Here's how the part is built. I have some questions about the finished solid (model axes, mm). Face numbers are marked on the shaded views. A direction names the side the tool comes from. Coordinates: 2 decimals unless noted, no trailing zeros. Loops run counter-clockwise (first coordinate to the right, second up) from the corner with the lowest first, then second, coordinate; pieces in that order, holes last. Notation, with made-up numbers: (6, -34.5) -> (11, -34.5) arc R26 cw to (11, -1.5) -> close; hole circle Ø10 at (42, -38.5). An arc over 180 degrees is marked (long way). Use CSV: the item, a comma, the result in double quotes. Start each with the question number.
from build123d import *

# Parameters (mm, degrees)
SKETCH1_W           = 127
SKETCH1_H           = 76.2
BOSS_EXTRUDE1_DEPTH = 76.2
CUT_EXTRUDE1_DEPTH  = 77.2
SKETCH3_W           = 58.776435242
SKETCH3_H           = 37.074512471
CUT_EXTRUDE2_DEPTH  = 77.2
SKETCH4_W           = 49.167351348
SKETCH4_H           = 86.931479723
BOSS_EXTRUDE3_DEPTH = 37.074512
CHAMFER1_SIZE       = 5.08
SKETCH5_R           = 3.175
BOSS_EXTRUDE4_DEPTH = 12.7
SKETCH6_W           = 49.167351348
SKETCH6_H           = 37.84167341
BOSS_EXTRUDE5_DEPTH = 5.08
SKETCH7_W           = 12.7
SKETCH7_H           = 3.957251341
BOSS_EXTRUDE6_DEPTH = 50.8
CHAMFER2_SIZE       = 4.445


with BuildPart() as part:
    # Sketch1 → Boss-Extrude1 (new body)
    with BuildSketch(Plane(origin=(0, 0, 0), x_dir=(1, 0, 0), z_dir=(0, 1, 0))):
        with Locations((63.5, 38.1)):
            Rectangle(SKETCH1_W, SKETCH1_H)
    extrude(amount=BOSS_EXTRUDE1_DEPTH)

    # Sketch2 → Cut-Extrude1 (cut, through all)
    with BuildSketch(Plane(origin=(0, 76.2, 0), x_dir=(1, 0, 0), z_dir=(0, 1, 0))):
        Polygon((86.341048303, 0), (105.391048303, 0), (105.391048303, 6.858), (111.233048303, 12.7), (80.499048303, 12.7), (86.341048303, 6.858), align=None)
    extrude(amount=-CUT_EXTRUDE1_DEPTH, mode=Mode.SUBTRACT)

    # Sketch3 → Cut-Extrude2 (cut, through all)
    with BuildSketch(Plane(origin=(0, 0, -76.2), x_dir=(-1, 0, 0), z_dir=(0, 0, -1))):
        with Locations((-29.388217621, 57.662743765)):
            Rectangle(SKETCH3_W, SKETCH3_H)
    extrude(amount=-CUT_EXTRUDE2_DEPTH, mode=Mode.SUBTRACT)

    # Sketch4 → Boss-Extrude3 (add)
    with BuildSketch(Plane(origin=(0, 39.125487529, 0), x_dir=(1, 0, 0), z_dir=(0, 1, 0))):
        with Locations((29.732558923, -5.365739861)):
            Rectangle(SKETCH4_W, SKETCH4_H)
    extrude(amount=BOSS_EXTRUDE3_DEPTH)

    # Chamfer1
    chamfer1_edges = [part.edges().sort_by_distance(p)[0] for p in [
        (5.148883249, 76.199999529, 5.365739861),
        (5.148883249, 39.125487529, 24.415739861),
        (54.316234597, 76.199999529, 5.365739861),
        (54.316234597, 39.125487529, 24.415739861),
    ]]
    chamfer(chamfer1_edges, length=CHAMFER1_SIZE)

    # Sketch5 → Boss-Extrude4 (add)
    with BuildSketch(Plane(origin=(0, 0, -38.1), x_dir=(-1, 0, 0), z_dir=(0, 0, -1))):
        with Locations((-45.312372158, 67.135265035)):
            Circle(SKETCH5_R)
        with Locations((-15.471955986, 67.135265035)):
            Circle(SKETCH5_R)
        with Locations((-45.312372158, 45.448629278)):
            Circle(SKETCH5_R)
        with Locations((-15.471955986, 45.448629278)):
            Circle(SKETCH5_R)
    extrude(amount=BOSS_EXTRUDE4_DEPTH)

    # Sketch6 → Boss-Extrude5 (add)
    with BuildSketch(Plane(origin=(0, 0, -50.8), x_dir=(-1, 0, 0), z_dir=(0, 0, -1))):
        with Locations((-29.732558923, 58.046324234)):
            Rectangle(SKETCH6_W, SKETCH6_H)
    extrude(amount=BOSS_EXTRUDE5_DEPTH)

    # Sketch7 → Boss-Extrude6 (add)
    with BuildSketch(Plane(origin=(0, 0, -55.88), x_dir=(-1, 0, 0), z_dir=(0, 0, -1))):
        with Locations((-40.016034597, 43.1361132)):
            Rectangle(SKETCH7_W, SKETCH7_H)
        with Locations((-19.365834597, 43.1361132)):
            Rectangle(SKETCH7_W, SKETCH7_H)
    extrude(amount=BOSS_EXTRUDE6_DEPTH)

    # Chamfer2
    chamfer2_edges = [part.edges().sort_by_distance(p)[0] for p in [
        (46.366034597, 43.1361132, -106.68),
        (33.666034597, 43.1361132, -106.68),
        (25.715834597, 43.1361132, -106.68),
        (13.015834597, 43.1361132, -106.68),
    ]]
    chamfer(chamfer2_edges, length=CHAMFER2_SIZE)


solid = part.part
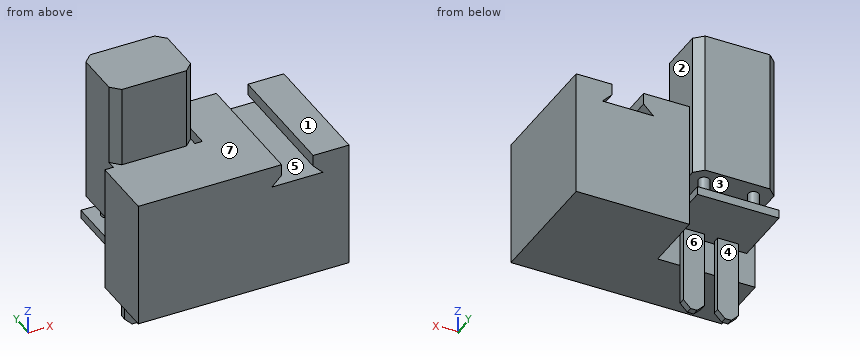
1) Which directions (+Z, -Z, +X, -X, +Y, -Y) give clear straight access to the entire face, cutting with the end or side of a thin tool? Please do the marked faces 1, 2, 3 and 4.
2) Please list where these lines run through material, in increasing order: L1, parallel to Z at x = 9, y = 48; L2, parallel to Y at x = 36.5, z = -67; L3, parallel to X at y = 31, z = -3.5. Write a range as [from, to].
3) I want a section at B-B, the plane y = 52.5. Please give me the cut outline in (x, z), plus the area to 3 significant figures.
4) I want a section at A-A, the plane z = -95.5. Please give me the cut outline in (x, y), plus the area to 3 significant figures.
5) Thinking about a two-plate mould opening in Z: for the marked faces 5, 6 and 7, which applies, pulls with the +Z half, pulls with the -Z half, needs draft (parallel to the pull), parting line crosses it, or undercut?
6) For P1, Ø1, axis at x = 97.5, y = 58, coming from the -Z side; P2, Ø2, axis at y = 42.5, z = -83.5, coming from the +X side; P3, Ø1, axis at x = 101, z = -69, coming from the +Y side; P4, Ø12, axis at y = 27.5, z = 25, coming from the +X side, each with a flat end and sliding along its axis, tell me the tip position at first contact or that it passes through.
7) I want a section at C-C, the plane z = -74. Please give me the cut outline in (x, y).
8) I want a section at D-D, the plane z = -41.5. Please give me the cut outline in (x, y) (3 decimals).
Return value:
1,face 1,"+Z, +X, +Y, -Y"
1,face 2,"+Z, -Z, +Y"
1,face 3,"none"
1,face 4,"-Z, -X, +Y"
2,L1,"z = [-55.88, -50.8], [-38.1, 48.83]"
2,L2,"y = [0, 39.13], [41.16, 45.11]"
2,L3,"x = [0, 86.34], [105.39, 127]"
3,outline,"(5.15, -55.88) -> (54.32, -55.88) -> (54.32, -50.8) -> (5.15, -50.8) -> close; (5.15, -38.1) -> (54.32, -38.1) -> (54.32, 48.83) -> (5.15, 48.83) -> close; (58.78, -76.2) -> (127, -76.2) -> (127, 0) -> (105.39, 0) -> (105.39, -6.86) -> (111.23, -12.7) -> (80.5, -12.7) -> (86.34, -6.86) -> (86.34, 0) -> (58.78, 0) -> close"
3,area,"9,450 mm²"
4,outline,"(13.02, 41.16) -> (25.72, 41.16) -> (25.72, 45.11) -> (13.02, 45.11) -> close; (33.67, 41.16) -> (46.37, 41.16) -> (46.37, 45.11) -> (33.67, 45.11) -> close"
4,area,"101 mm²"
5,face 5,"undercut"
5,face 6,"needs draft"
5,face 7,"pulls with the +Z half"
6,P1,"stops at z = -76.2"
6,P2,"stops at x = 46.37"
6,P3,"stops at y = 76.2"
6,P4,"passes through"
7,outline,"(0, 0) -> (127, 0) -> (127, 76.2) -> (58.78, 76.2) -> (58.78, 39.13) -> (0, 39.13) -> close; (13.02, 41.16) -> (25.72, 41.16) -> (25.72, 45.11) -> (13.02, 45.11) -> close; (33.67, 41.16) -> (46.37, 41.16) -> (46.37, 45.11) -> (33.67, 45.11) -> close"
8,outline,"(0, 0) -> (127, 0) -> (127, 76.2) -> (58.776, 76.2) -> (58.776, 39.125) -> (0, 39.125) -> close; circle Ø6.35 at (15.472, 45.449); circle Ø6.35 at (15.472, 67.135); circle Ø6.35 at (45.312, 45.449); circle Ø6.35 at (45.312, 67.135)"
